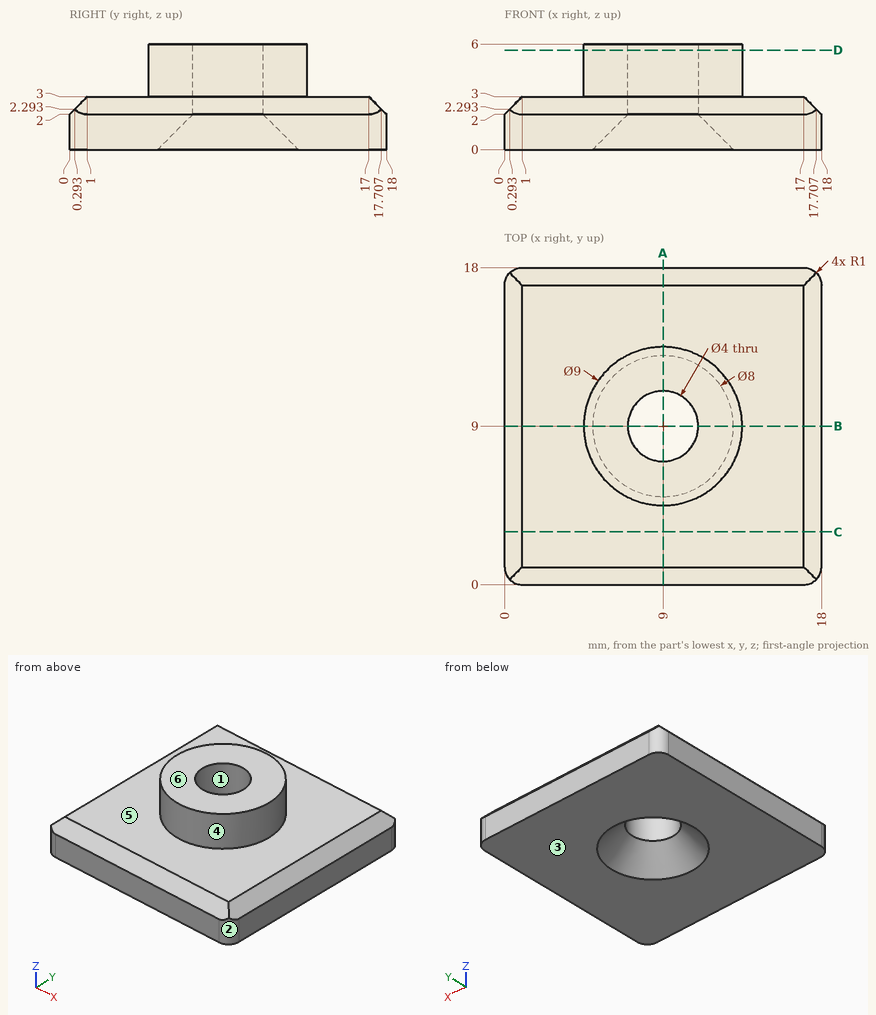
Input: dimensioned drawing with shaded views. Units: mm. Origin: part minimum x, y, z. A direction names the side the tool comes from. Round coordinates to 2 decimals unless told otherwise and drop trailing zeros. Loops run counter-clockwise (first coordinate to the right, second up) from the corner with the lowest first, then second, coordinate; pieces in that order, holes last. Notation, with made-up numbers: M -0.75,23.5 L 11.25,23.5 A24 cw 11.25,43.5 Z; hole C 55,50.5 d1. An arc over 180 degrees is marked long. One line per question, with ' | ' between items.
(1) Pull-direction query (Y, two-part tool) for the marked faces 1, 2, 3 and 4; classes: +Y half, -Y half, draft (parallel to the pull), parting line (faces both ways), or undercut.
Check result:
face 1: undercut | face 2: -Y half | face 3: draft | face 4: parting line
(2) Cut plane C-C on y = 3. Return the cut outline in (x, z).
Check result:
outline: M 0,0 L 18,0 L 18,2 L 17,3 L 1,3 L 0,2 Z
(3) Contact query for a flat-ended pin moving along its axis: P1, Ø2.5, axis at x = 9, y = 9, coming from the -Z side. Output: stop coordinate, or through.
Check result:
P1: passes through
(4) Material intervals for line 1 along Y through (x, z) = (9, 3.15); line 2 along Z through (x, y) = (15, 12.5); line 3 along Y through (x, z) = (7, 1.5), sorted ascending. Write a range as from..to.
Check result:
line 1: y = 4.5..7, 11..13.5 | line 2: z = 0..3 | line 3: y = 0..7.5, 10.5..18
(5) Cut plane D-D on z = 5.65. Return the cut outline in (x, y).
Check result:
outline: C 9,9 d9; hole C 9,9 d4
(6) Access query for the marked faces 5 and 6. Directions: +Z, -Z, +X, -X, +Y, -Y. A direction counts if a zero-diameter tool reaches every point of the face in a straight line with its end or side. Return the directions, or none.
Check result:
face 5: +Z | face 6: +Z, +X, -X, +Y, -Y
(7) Cut plane A-A on x = 9. Return the cut outline in (y, z), plus the area to 3 significant figures.
Check result:
outline: M 0,0 L 5,0 L 7,2 L 7,6 L 4.5,6 L 4.5,3 L 1,3 L 0,2 Z; M 11,2 L 13,0 L 18,0 L 18,2 L 17,3 L 13.5,3 L 13.5,6 L 11,6 Z | area: 52.0 mm2
